from build123d import *

# Parameters (mm, degrees)
SKETCH1_R            = 1
BOSS_EXTRUDE1_DEPTH  = 12
CUT_EXTRUDE1_DEPTH   = 4.25
CUT_EXTRUDE3_DEPTH   = 4.25
CUT_EXTRUDE2_START   = -3.551923789
CUT_EXTRUDE2_DEPTH   = 3.551923789
CUT_EXTRUDE2_START_2 = 4.25
CUT_EXTRUDE2_2_DEPTH = 3.5
FILLET8_R            = 1
FILLET9_R            = 1


with BuildPart() as part:
    # Sketch1 → Boss-Extrude1 (new body)
    with BuildSketch(Plane.XY):
        with BuildLine():
            Line((1.186636508, 7.015339144), (10.241749958, 13.764812698))
            ThreePointArc((10.241749958, 13.764812698), (10.336328118, 16.101061111), (11.720750751, 17.985305164))
            ThreePointArc((11.720750751, 17.985305164), (12.854265392, 17.819943261), (12.688903489, 16.68642862))
            ThreePointArc((12.688903489, 16.68642862), (12.203025305, 13.355854737), (15.533599188, 12.869976553))
            ThreePointArc((15.533599188, 12.869976553), (16.667113829, 12.704614651), (16.501751927, 11.57110001))
            ThreePointArc((16.501751927, 11.57110001), (14.300524873, 10.782683155), (12.034625399, 11.359485765))
            Line((12.034625399, 11.359485765), (2.979511949, 4.610012211))
            ThreePointArc((2.979511949, 4.610012211), (2.843457612, 3.303574986), (2.162315925, 2.180483268))
            Line((2.162315925, 2.180483268), (5.498303396, 3.137062282))
            Line((5.498303396, 3.137062282), (6.325215464, 0.253277194))
            Line((6.325215464, 0.253277194), (6.880438917, -1.683017096))
            Line((6.880438917, -1.683017096), (6.052988912, -1.920284566))
            Line((6.052988912, -1.920284566), (3.421928238, -0.579227021))
            Line((3.421928238, -0.579227021), (2.910887179, -0.725765687))
            ThreePointArc((2.910887179, -0.725765687), (-1.48262032, -2.608033164), (-2.112605027, 2.13))
            ThreePointArc((-2.112605027, 2.13), (-2.486159501, 5.938991047), (1.186636508, 7.015339144))
        make_face()
        with Locations((0, 4.26)):
            Circle(SKETCH1_R, mode=Mode.SUBTRACT)
        Circle(SKETCH1_R, mode=Mode.SUBTRACT)
    extrude(amount=BOSS_EXTRUDE1_DEPTH)

    # Sketch2 → Cut-Extrude1 (cut)
    with BuildSketch(Plane.XY.offset(12)):
        with BuildLine():
            ThreePointArc((2.520535657, 2.13), (0, 7.56), (-2.520535657, 2.13))
            ThreePointArc((-2.520535657, 2.13), (0, -3.3), (2.520535657, 2.13))
        make_face()
    cut_extrude1 = extrude(amount=-CUT_EXTRUDE1_DEPTH, mode=Mode.SUBTRACT)

    # Sketch4 → Cut-Extrude3 (cut)
    with BuildSketch(Plane.XY.offset(12)):
        Polygon((7.542328095, 11.752725651), (9.335203536, 9.347398719), (2.498013424, 4.251114272), (0.705137983, 6.656441205), align=None)
    cut_extrude3 = extrude(amount=-CUT_EXTRUDE3_DEPTH, mode=Mode.SUBTRACT)

    # Mirror1: Cut-Extrude1, Cut-Extrude3 across plane
    add(cut_extrude1.mirror(Plane.XY.offset(6)), mode=Mode.SUBTRACT)
    add(cut_extrude3.mirror(Plane.XY.offset(6)), mode=Mode.SUBTRACT)

    # Cut-Extrude2: read off the stored shape, not the designer's step
    # Cut-Extrude2 outline → Cut-Extrude2 (cut)
    with BuildSketch(Plane(origin=(5.91175943, 1.695169738, 0), x_dir=(0, 0, -1), z_dir=(0.9612616959383197, 0.27563735581699633, 0)).offset(CUT_EXTRUDE2_START)):
        Polygon((0, 1.5), (-12, -3.514325857), (0, -3.514325857), align=None)
    extrude(amount=CUT_EXTRUDE2_DEPTH, mode=Mode.SUBTRACT)

    # Cut-Extrude2 2 outline → Cut-Extrude2 2 (add)
    with BuildSketch(Plane.XY.offset(CUT_EXTRUDE2_START_2)):
        with BuildLine():
            ThreePointArc((2.910887178, -0.725765687), (2.998773461, -0.085777187), (2.947613523, 0.558188603))
            Line((2.947613523, 0.558188603), (2.674578173, 2))
            Line((2.674578173, 2), (2.129286445, 2))
            Line((2.129286445, 2), (2.573481441, 0.450907955))
            Line((2.573481441, 0.450907955), (2.910887178, -0.725765687))
        make_face()
    extrude(amount=CUT_EXTRUDE2_2_DEPTH)

    # Fillet8
    fillet8_edges = [part.edges().sort_by_distance(p)[0] for p in [
        (10.241749958, 13.764812698, 6),
        (12.034625399, 11.359485765, 6),
    ]]
    fillet(fillet8_edges, radius=FILLET8_R)

    # Fillet9
    fillet9_edges = [part.edges().sort_by_distance(p)[0] for p in [
        (6.189371157, 0.727022594, 6),
    ]]
    fillet(fillet9_edges, radius=FILLET9_R)


solid = part.part
Geometry check sheet. Reference: the model listing, model coordinates, mm. A direction names the side the tool comes from. Round coordinates to 2 decimals unless told otherwise and drop trailing zeros. Loops run counter-clockwise (first coordinate to the right, second up) from the corner with the lowest first, then second, coordinate; pieces in that order, holes last.
Item 1: Cross-section at C-C on x = 9. Record the boundary of the cut face in (y, z).
Item 2: Cross-section at B-B on x = 0. Record the boundary of the cut face in (y, z).
Item 3: Gauge pin test, flat ends, axial feed: pin 1 (3 mm diameter, centred on y = 15, z = 9, fed in from +X); pin 2 (2 mm diameter, centred on x = 8.5, z = 10.5, fed in from +Y); pin 3 (8 mm diameter, centred on x = 2, y = 13.5, fed in from -Z); pin 4 (2.5 mm diameter, centred on x = 0, y = 0, fed in from +Z). Record the tip position at first contact, or that the pin passes through.
Item 4: Thickness scan on line 1 (Y direction, x = 0, z = 6.7); line 2 (X direction, y = 4.26, z = 6.45); line 3 (Z direction, x = 1.75, y = -0.25). Record the ranges inside material, lowest first.
Item 5: Cross-section at A-A on y = 4.26. Record the boundary of the cut face in (x, z), then the cut area to 3 significant figures.
Item 6: Access from +Z, -Z, +X, -X, +Y, -Y to the whole of each face (thin tool, end or side, straight path). Record for faces 4 (the cylindrical face through (3.2, 0.8, 9.9)), 5 (the cylindrical face through (2.8, 1.75, 3.14)), 6 (the flat face through (8.4, 10.6, 9.9)).
Item 7: Cross-section at D-D on z = 6.75. Count the separate pieces of the cut face and the enclosed holes in it, then the cut area to 3 significant figures.
Item 8: Mould release check, pull along Y, two halves, no side actions. Record for faces 1 (the flat face through (12, 12, 0)), 2 (the cylindrical face through (12.01, 11.18, 6.08)), 3 (the flat face through (3.807, 2.652, 5.916)): pulls with the +Y half, pulls with the -Y half, needs draft (parallel to the pull), parting line crosses it, or undercut.
Answer sheet:
1. outline: (9.1, 4.25) - (9.8, 4.25) - (9.8, 0) - (12.84, 0) - (12.84, 12) - (9.8, 12) - (9.8, 7.75) - (9.1, 7.75) - close
2. outline: (-3, 4.25) - (-1, 4.25) - (-1, 7.75) - (-3, 7.75) - close; (1, 4.25) - (3.26, 4.25) - (3.26, 7.75) - (1, 7.75) - close; (5.26, 4.25) - (7.26, 4.25) - (7.26, 7.75) - (5.26, 7.75) - close
3. pin 1: stops at x = 12.47
3. pin 2: stops at y = 13.21
3. pin 3: passes through
3. pin 4: stops at z = 7.75
4. line 1: y = -3 to -1, 1 to 3.26, 5.26 to 7.26
4. line 2: x = -3 to -1, 1 to 3
4. line 3: z = 4.25 to 7.75
5. outline: (-3, 4.25) - (-1, 4.25) - (-1, 7.75) - (-3, 7.75) - close; (1, 4.25) - (3, 4.25) - (3, 7.75) - (1, 7.75) - close
5. area: 14.0 mm2
6. face 4: +Z, -X
6. face 5: -Z, -X, -Y
6. face 6: +Z, -X, -Y
7. separate pieces: 1
7. enclosed holes: 2
7. area: 105 mm2
8. face 1: needs draft
8. face 2: pulls with the -Y half
8. face 3: undercut
